```python
from build123d import *

# Parameters (mm, degrees)
SKETCH1_W           = 144
SKETCH1_H           = 80
BOSS_EXTRUDE1_DEPTH = 50
CUT_EXTRUDE1_REACH  = 98.354
SKETCH2_R           = 10
SKETCH2_R_2         = 13
CUT_EXTRUDE3_REACH  = 98.354
SKETCH3_W           = 144
SKETCH3_H           = 20
SKETCH5_R           = 3
CUT_EXTRUDE4_DEPTH  = 100
FILLET1_R           = 10
FILLET2_R           = 10
FILLET3_R           = 10
FILLET4_R           = 10
SKETCH6_R           = 5.5
CUT_EXTRUDE5_DEPTH  = 5
SKETCH7_W           = 30
SKETCH7_H           = 40
BOSS_EXTRUDE2_DEPTH = 10
CUT_EXTRUDE7_REACH  = 108.226
SKETCH8_R           = 3


with BuildPart() as part:
    # Sketch1 → Boss-Extrude1 (new body)
    with BuildSketch(Plane.XY):
        Rectangle(SKETCH1_W, SKETCH1_H)
    extrude(amount=BOSS_EXTRUDE1_DEPTH)

    # Sketch2 → Cut-Extrude1 (cut, up to next)
    with BuildSketch(Plane.XY.offset(50), mode=Mode.PRIVATE) as cut_extrude1_sk1:
        Circle(SKETCH2_R)
    cut_extrude1_tool1 = extrude(cut_extrude1_sk1.sketch, amount=-CUT_EXTRUDE1_REACH, mode=Mode.PRIVATE) & part.part
    # Sketch2 → Cut-Extrude1 (cut, up to next)
    with BuildSketch(Plane.XY.offset(50), mode=Mode.PRIVATE) as cut_extrude1_sk2:
        with Locations((-50, 0)):
            Circle(SKETCH2_R_2)
    cut_extrude1_tool2 = extrude(cut_extrude1_sk2.sketch, amount=-CUT_EXTRUDE1_REACH, mode=Mode.PRIVATE) & part.part
    # Sketch2 → Cut-Extrude1 (cut, up to next)
    with BuildSketch(Plane.XY.offset(50), mode=Mode.PRIVATE) as cut_extrude1_sk3:
        with Locations(Location((50, 0, 0), (0, 0, 180))):
            Circle(SKETCH2_R_2)
    cut_extrude1_tool3 = extrude(cut_extrude1_sk3.sketch, amount=-CUT_EXTRUDE1_REACH, mode=Mode.PRIVATE) & part.part
    add(cut_extrude1_tool1.solids().sort_by_distance((0, 0, 50))[0], mode=Mode.SUBTRACT)
    add(cut_extrude1_tool2.solids().sort_by_distance((-50, 0, 50))[0], mode=Mode.SUBTRACT)
    add(cut_extrude1_tool3.solids().sort_by_distance((50, 0, 50))[0], mode=Mode.SUBTRACT)

    # Sketch3 → Cut-Extrude3 (cut, up to next)
    with BuildSketch(Plane.XY.offset(50), mode=Mode.PRIVATE) as cut_extrude3_sk1:
        with Locations((0, -30)):
            Rectangle(SKETCH3_W, SKETCH3_H)
    cut_extrude3_tool1 = extrude(cut_extrude3_sk1.sketch, amount=-CUT_EXTRUDE3_REACH, mode=Mode.PRIVATE) & part.part
    add(cut_extrude3_tool1.solids().sort_by_distance((0, -30, 50))[0], mode=Mode.SUBTRACT)

    # Sketch5 → Cut-Extrude4 (cut)
    with BuildSketch(Plane.XZ.offset(20)):
        with Locations(Location((-22, 34, 0), (0, 0, 270))):
            Circle(SKETCH5_R)
        with Locations(Location((-22, 14, 0), (0, 0, 270))):
            Circle(SKETCH5_R)
    extrude(amount=-CUT_EXTRUDE4_DEPTH, mode=Mode.SUBTRACT)

    # Fillet1
    fillet1_edges = [part.edges().sort_by_distance(p)[0] for p in [
        (72, -20, 25),
    ]]
    fillet(fillet1_edges, radius=FILLET1_R)

    # Fillet2
    fillet2_edges = [part.edges().sort_by_distance(p)[0] for p in [
        (72, 40, 25),
    ]]
    fillet(fillet2_edges, radius=FILLET2_R)

    # Fillet3
    fillet3_edges = [part.edges().sort_by_distance(p)[0] for p in [
        (-72, 40, 25),
    ]]
    fillet(fillet3_edges, radius=FILLET3_R)

    # Fillet4
    fillet4_edges = [part.edges().sort_by_distance(p)[0] for p in [
        (-72, -20, 25),
    ]]
    fillet(fillet4_edges, radius=FILLET4_R)

    # Sketch6 → Cut-Extrude5 (cut)
    with BuildSketch(Plane(origin=(0, 40, 0), x_dir=(1, 0, 0), z_dir=(0, 1, 0))):
        with Locations(Location((-22, -14, 0), (0, 0, 270))):
            Circle(SKETCH6_R)
        with Locations(Location((-22, -34, 0), (0, 0, 270))):
            Circle(SKETCH6_R)
    extrude(amount=-CUT_EXTRUDE5_DEPTH, mode=Mode.SUBTRACT)

    # Sketch7 → Boss-Extrude2 (add)
    with BuildSketch(Plane.XZ.offset(20)):
        with Locations((-22, 25)):
            Rectangle(SKETCH7_W, SKETCH7_H)
    extrude(amount=BOSS_EXTRUDE2_DEPTH)

    # Sketch8 → Cut-Extrude7 (cut, up to next)
    with BuildSketch(Plane(origin=(0, -20, 0), x_dir=(1, 0, 0), z_dir=(0, 1, 0)), mode=Mode.PRIVATE) as cut_extrude7_sk1:
        with Locations(Location((-22, -34, 0), (0, 0, 90))):
            Circle(SKETCH8_R)
    cut_extrude7_tool1 = extrude(cut_extrude7_sk1.sketch, amount=-CUT_EXTRUDE7_REACH, mode=Mode.PRIVATE) & part.part
    # Sketch8 → Cut-Extrude7 (cut, up to next)
    with BuildSketch(Plane(origin=(0, -20, 0), x_dir=(1, 0, 0), z_dir=(0, 1, 0)), mode=Mode.PRIVATE) as cut_extrude7_sk2:
        with Locations(Location((-22, -14, 0), (0, 0, 90))):
            Circle(SKETCH8_R)
    cut_extrude7_tool2 = extrude(cut_extrude7_sk2.sketch, amount=-CUT_EXTRUDE7_REACH, mode=Mode.PRIVATE) & part.part
    add(cut_extrude7_tool1.solids().sort_by_distance((-22, -20, 34))[0], mode=Mode.SUBTRACT)
    add(cut_extrude7_tool2.solids().sort_by_distance((-22, -20, 14))[0], mode=Mode.SUBTRACT)


solid = part.part
```
Design review of the part built by this model. Coordinates are the model's own, in mm. A direction names the side the tool comes from. Coordinates: 2 decimals unless noted, no trailing zeros. Write each loop counter-clockwise with the first axis right and the second up, starting at its lowest first coordinate (ties: lowest second). Pieces come first, ordered by that corner, then holes.
1) Add section A-A (z = 34). Write out the cut boundary in (x, y), plus the area to 3 significant figures.
2) Machinability: for faces 4 (the flat face through (-22, -25, 45)), 5 (the cylindrical face through (-68.99, 37.15, 25.35)), 6 (the flat face through (-24.4, 35, 16.4)), 7 (the flat face through (-7, -25, 25)), 8 (the flat face through (-37, -25, 25)), which of the approach directions +Z, -Z, +X, -X, +Y, -Y give a long, thin tool a straight path to every point of the face, cutting with its end or side? Answer none if there is none.
3) Add section D-D (y = -2). Write out the cut boundary in (x, z).
4) Add section C-C (z = 22). Write out the cut boundary in (x, y).
5) To check wall thickness, follow L1, parallel to Z at x = -22, y = 3; L2, parallel to Y at x = -50, z = 24; L3, parallel to Y at x = 0, z = 36. State the ranges of each line that lie inside material, in increasing order.
6) Insertion check: pin 1 (5.5 mm diameter, centred on x = -23.5, z = 15, fed in from +Y); pin 2 (5 mm diameter, centred on x = -21.5, y = -23.5, fed in from +Z); pin 3 (8 mm diameter, centred on x = -28.5, y = -25, fed in from -Z); pin 4 (15.5 mm diameter, centred on x = -50, y = 0, fed in from +Z). Each pin has a flat end and moves straight along its axis. Give the tip position at first contact, or say it passes through.
7) Add section B-B (x = 0). Write out the cut boundary in (y, z).
8) Mouldability with a two-part tool opening along X and no side actions: class faces 1 (the flat face through (72, 10, 25)), 2 (the flat face through (-22, -25, 5)), 3 (the cylindrical face through (-2.17, -9.76, 25.35)) as +X half, -X half, draft (parallel to the pull), parting line (faces both ways), or undercut.
Check result:
1. outline: (-72, -10) arc R10 ccw to (-62, -20) - (-37, -20) - (-37, -30) - (-25, -30) - (-25, 35) - (-27.5, 35) - (-27.5, 40) - (-62, 40) arc R10 ccw to (-72, 30) - close; (-19, -30) - (-7, -30) - (-7, -20) - (62, -20) arc R10 ccw to (72, -10) - (72, 30) arc R10 ccw to (62, 40) - (-16.5, 40) - (-16.5, 35) - (-19, 35) - close; hole circle Ø26 at (-50, 0); hole circle Ø20 at (0, 0); hole circle Ø26 at (50, 0)
1. area: 7,030 mm2
2. face 4: +Z, +X, -X, -Y
2. face 5: +Z, -Z, -X, +Y
2. face 6: +Y
2. face 7: +Z, -Z, +X, -Y
2. face 8: +Z, -Z, -X, -Y
3. outline: (-72, 0) - (-62.85, 0) - (-62.85, 50) - (-72, 50) - close; (-37.15, 0) - (-9.8, 0) - (-9.8, 50) - (-37.15, 50) - close; (9.8, 0) - (37.15, 0) - (37.15, 50) - (9.8, 50) - close; (62.85, 0) - (72, 0) - (72, 50) - (62.85, 50) - close; hole circle Ø6 at (-22, 14); hole circle Ø6 at (-22, 34)
4. outline: (-72, -10) arc R10 ccw to (-62, -20) - (-37, -20) - (-37, -30) - (-7, -30) - (-7, -20) - (62, -20) arc R10 ccw to (72, -10) - (72, 30) arc R10 ccw to (62, 40) - (-62, 40) arc R10 ccw to (-72, 30) - close; hole circle Ø26 at (-50, 0); hole circle Ø20 at (0, 0); hole circle Ø26 at (50, 0)
5. L1: z = 0 to 11, 17 to 31, 37 to 50
5. L2: y = -20 to -13, 13 to 40
5. L3: y = -20 to -10, 10 to 40
6. pin 1: stops at y = 35
6. pin 2: stops at z = 45
6. pin 3: stops at z = 5
6. pin 4: passes through
7. outline: (-20, 0) - (-10, 0) - (-10, 50) - (-20, 50) - close; (10, 0) - (40, 0) - (40, 50) - (10, 50) - close
8. face 1: +X half
8. face 2: draft
8. face 3: undercut
